Check sheet for the modelled part. Datum: model origin and axes. Units: mm. A direction names the side the tool comes from. Round coordinates to 2 decimals unless told otherwise and drop trailing zeros. Write each loop counter-clockwise with the first axis right and the second up, starting at its lowest first coordinate (ties: lowest second). Pieces come first, ordered by that corner, then holes.
Item 1: Cross-section at A-A on x = 698.5. Enter the section's corners in (y, z) (3 decimals), plus the area to 3 significant figures.
Item 2: Cross-section at C-C on z = 6.5. Enter the section's corners in (x, y) (3 decimals), plus the area to 3 significant figures.
Item 3: Cross-section at B-B on y = 0. Enter the section's corners in (x, z) (3 decimals), plus the area to 3 significant figures.
Item 4: Material ranges on line 1 (Z direction, x = 437, y = -9) (3 decimals); line 2 (Y direction, x = 12.7, z = 18.2), recorded low to high.
Item 5: Release check for a two-part mould opening along X. For faces 3 (the cylindrical face through (704.557, 1.907, 17.485)), 4 (the flat face through (711.2, -17, 0)), 5 (the flat face through (351, 19.05, 0)) record: +X half, -X half, draft (parallel to the pull), parting line (faces both ways), or undercut.
Item 6: Cross-section at D-D on x = 604.5. Enter the section's corners in (y, z) (3 decimals).
Item 7: Go/stop test with flat-tipped pins: pin 1 Ø20.5 at (x, y) = (12.7, 0) entering from -Z; pin 2 Ø1.5 at (x, y) = (280, -15) entering from +Z; pin 3 Ø1.5 at (y, z) = (13.5, -3.5) entering from -X. Record where each tip stops, or that it passes through.
Item 8: Tool access check on faces 1 (the flat face through (351, 0, 19.05)), 2 (the flat face through (351, 0, 15.875)). Record the directions out of +Z, -Z, +X, -X, +Y, -Y that give a thin tool (end or side, any length) a straight path to the whole face; none if there is none.
from build123d import *

# Parameters (mm, degrees)
STRUCTURAL_MEMBER1_DEPTH = 711.2
SKETCH2_R                = 6.35
CUT_EXTRUDE1_DEPTH       = 713.474527615
SKETCH3_R                = 6.35
CUT_EXTRUDE2_DEPTH       = 713.474527615


with BuildPart() as part:
    # Sketch1 → Structural Member1 (new body)
    with BuildSketch(Plane(origin=(0, 0, 0), x_dir=(0, 0, -1), z_dir=(1, 0, 0))):
        with BuildLine():
            Line((-12.7, -19.05), (12.7, -19.05))
            ThreePointArc((12.7, -19.05), (17.190128061, -17.190128061), (19.05, -12.7))
            Line((19.05, -12.7), (19.05, 12.7))
            ThreePointArc((19.05, 12.7), (17.190128061, 17.190128061), (12.7, 19.05))
            Line((12.7, 19.05), (-12.7, 19.05))
            ThreePointArc((-12.7, 19.05), (-17.190128061, 17.190128061), (-19.05, 12.7))
            Line((-19.05, 12.7), (-19.05, -12.7))
            ThreePointArc((-19.05, -12.7), (-17.190128061, -17.190128061), (-12.7, -19.05))
        make_face()
        with BuildLine():
            Line((-12.7, -15.875), (12.7, -15.875))
            ThreePointArc((12.7, -15.875), (14.94506403, -14.94506403), (15.875, -12.7))
            Line((15.875, -12.7), (15.875, 12.7))
            ThreePointArc((15.875, 12.7), (14.94506403, 14.94506403), (12.7, 15.875))
            Line((12.7, 15.875), (-12.7, 15.875))
            ThreePointArc((-12.7, 15.875), (-14.94506403, 14.94506403), (-15.875, 12.7))
            Line((-15.875, 12.7), (-15.875, -12.7))
            ThreePointArc((-15.875, -12.7), (-14.94506403, -14.94506403), (-12.7, -15.875))
        make_face(mode=Mode.SUBTRACT)
    extrude(amount=STRUCTURAL_MEMBER1_DEPTH)

    # Sketch2 → Cut-Extrude1 (cut, through all)
    with BuildSketch(Plane.XY.offset(19.05)):
        with Locations((12.7, 0)):
            Circle(SKETCH2_R)
    extrude(amount=-CUT_EXTRUDE1_DEPTH, mode=Mode.SUBTRACT)

    # Sketch3 → Cut-Extrude2 (cut, through all)
    with BuildSketch(Plane.XY.offset(19.05)):
        with Locations((698.5, 0)):
            Circle(SKETCH3_R)
    extrude(amount=-CUT_EXTRUDE2_DEPTH, mode=Mode.SUBTRACT)


solid = part.part
Response values:
1. outline: (-19.05, -12.7) arc R6.35 ccw to (-12.7, -19.05) - (-6.35, -19.05) - (-6.35, -15.875) - (-12.7, -15.875) arc R3.175 cw to (-15.875, -12.7) - (-15.875, 12.7) arc R3.175 cw to (-12.7, 15.875) - (-6.35, 15.875) - (-6.35, 19.05) - (-12.7, 19.05) arc R6.35 ccw to (-19.05, 12.7) - close; (6.35, -19.05) - (12.7, -19.05) arc R6.35 ccw to (19.05, -12.7) - (19.05, 12.7) arc R6.35 ccw to (12.7, 19.05) - (6.35, 19.05) - (6.35, 15.875) - (12.7, 15.875) arc R3.175 cw to (15.875, 12.7) - (15.875, -12.7) arc R3.175 cw to (12.7, -15.875) - (6.35, -15.875) - close
1. area: 337 mm2
2. outline: (0, -19.05) - (711.2, -19.05) - (711.2, -15.875) - (0, -15.875) - close; (0, 15.875) - (711.2, 15.875) - (711.2, 19.05) - (0, 19.05) - close
2. area: 4,520 mm2
3. outline: (0, -19.05) - (6.35, -19.05) - (6.35, -15.875) - (0, -15.875) - close; (0, 15.875) - (6.35, 15.875) - (6.35, 19.05) - (0, 19.05) - close; (19.05, -19.05) - (692.15, -19.05) - (692.15, -15.875) - (19.05, -15.875) - close; (19.05, 15.875) - (692.15, 15.875) - (692.15, 19.05) - (19.05, 19.05) - close; (704.85, -19.05) - (711.2, -19.05) - (711.2, -15.875) - (704.85, -15.875) - close; (704.85, 15.875) - (711.2, 15.875) - (711.2, 19.05) - (704.85, 19.05) - close
3. area: 4,350 mm2
4. line 1: z = -19.05 to -15.875, 15.875 to 19.05
4. line 2: y = -15.87 to -6.35, 6.35 to 15.87
5. face 3: undercut
5. face 4: +X half
5. face 5: draft
6. outline: (-19.05, -12.7) arc R6.35 ccw to (-12.7, -19.05) - (12.7, -19.05) arc R6.35 ccw to (19.05, -12.7) - (19.05, 12.7) arc R6.35 ccw to (12.7, 19.05) - (-12.7, 19.05) arc R6.35 ccw to (-19.05, 12.7) - close; hole (-15.875, -12.7) arc R3.175 ccw to (-12.7, -15.875) - (12.7, -15.875) arc R3.175 ccw to (15.875, -12.7) - (15.875, 12.7) arc R3.175 ccw to (12.7, 15.875) - (-12.7, 15.875) arc R3.175 ccw to (-15.875, 12.7) - close
7. pin 1: stops at z = -19.05
7. pin 2: stops at z = 18.86
7. pin 3: passes through
8. face 1: +Z, +X, -X, +Y, -Y
8. face 2: +X, -X
